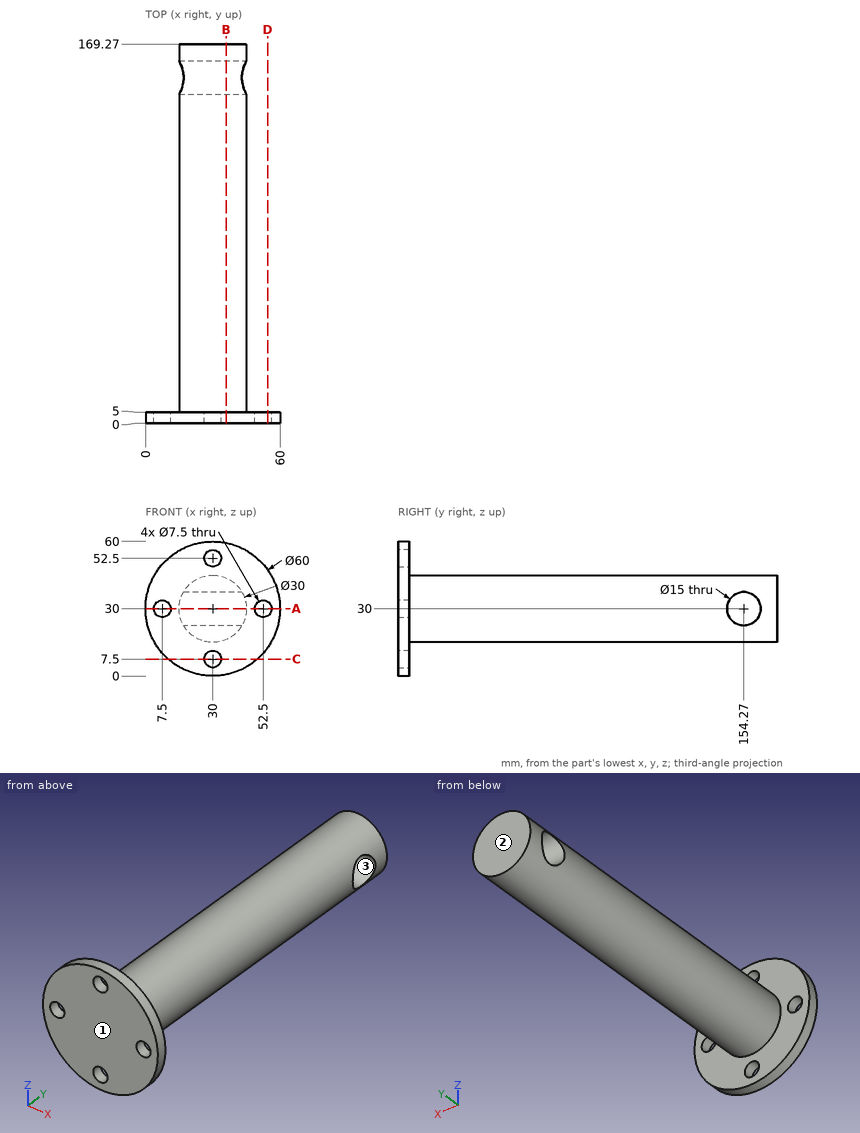
Could you check a few things on this drawing? It's one solid part, dimensions in mm from its lowest x, y, z. Give positions to 0.01 mm unless a question says otherwise; leave off trailing zeros. Order: outer loops, then holes, each group sorted by start corner. A loop starts at its lowest first (then second) coordinate and runs counter-clockwise, first axis right, second up. Notation, with made-up numbers: M 79.25,89 L 103.25,89 A9 cw 103.25,100 Z; hole C 7,14 d3. An arc over 180 degrees is marked long. Use one line per item in the form item = value. Start each with the question number.
Item 1: Will these pins go through, and if not, where does the flat tip stop? pin 1 Ø8.5 at (x, z) = (30, 52.5) entering from -Y; pin 2 Ø12 at (x, z) = (52.5, 30) entering from +Y; pin 3 Ø6 at (y, z) = (80, 13.5) entering from +X; pin 4 Ø3 at (y, z) = (54.5, 16) entering from -X.
Item 2: If we section it at B-B (x = 36): Write out the boundary of the cut face in (y, z).
Item 3: If we section it at D-D (x = 54.5): Write out the boundary of the cut face in (y, z), then the cut area to 3 significant figures.
Item 4: If I drill on line 1 along X through (y, z) = (3.7, 30); line 2 along Y through (x, z) = (53, 16.5); line 3 along Z through (x, y) = (52, 1), over which ranges is the centre line in solid material (lowest first)?
Item 5: We'd pull the mould along Y, two halves only. Please class the marked faces 1, 2 and 3: +Y half, -Y half, draft (parallel to the pull), parting line (faces both ways), or undercut.
Item 6: If we section it at C-C (z = 7.5): Write out the boundary of the cut face in (x, y).
Item 7: If we section it at A-A (z = 30): Write out the boundary of the cut face in (x, y).
Outcome:
q1.pin_1 = 0
q1.pin_2 = 5
q1.pin_3 = 36.54
q1.pin_4 = 21.71
q2.outline = M 0,0.61 L 5,0.61 L 5,16.25 L 169.27,16.25 L 169.27,43.75 L 5,43.75 L 5,59.39 L 0,59.39 Z; hole C 154.27,30 d15
q3.outline = M 0,12.69 L 5,12.69 L 5,26.83 L 0,26.83 Z; M 0,33.17 L 5,33.17 L 5,47.31 L 0,47.31 Z
q3.area = 141 mm2
q4.line_1 = 0 to 3.75, 11.25 to 48.75, 56.25 to 60
q4.line_2 = 0 to 5
q4.line_3 = 9.6 to 26.28, 33.72 to 50.4
q5.face_1 = -Y half
q5.face_2 = +Y half
q5.face_3 = undercut
q6.outline = M 10.16,0 L 26.25,0 L 26.25,5 L 10.16,5 Z; M 33.75,0 L 49.84,0 L 49.84,5 L 33.75,5 Z
q7.outline = M 0,0 L 3.75,0 L 3.75,5 L 0,5 Z; M 11.25,0 L 48.75,0 L 48.75,5 L 45,5 L 45,146.77 L 15,146.77 L 15,5 L 11.25,5 Z; M 15,161.77 L 45,161.77 L 45,169.27 L 15,169.27 Z; M 56.25,0 L 60,0 L 60,5 L 56.25,5 Z
